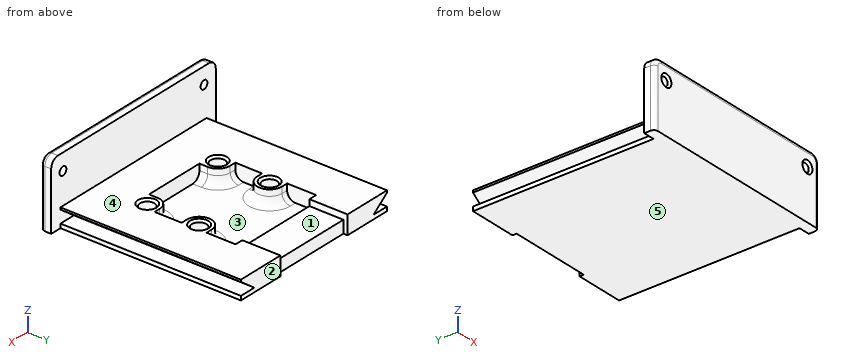
```python
from build123d import *

# Parameters (mm, degrees)
ESQUISSE1_W             = 43.5
ESQUISSE1_H             = 43.5
BOSS_EXTRU_1_DEPTH      = 3.5
ESQUISSE3_W             = 24
ESQUISSE3_H             = 24.5
ENL_V_MAT_EXTRU_1_DEPTH = 3.5
ENL_V_MAT_EXTRU_3_DEPTH = 43.5
ESQUISSE5_W             = 20
ESQUISSE5_H             = 9.18
ENL_V_MAT_EXTRU_4_DEPTH = 1.5
BOSS_EXTRU_2_DEPTH      = 3.5
ESQUISSE8_R             = 1.75
ENL_V_MAT_EXTRU_5_DEPTH = 3.5
ESQUISSE9_W             = 43.5
ESQUISSE9_H             = 43.5
BOSS_EXTRU_3_DEPTH      = 1
CONG_2_R                = 2
CHANFREIN1_SIZE         = 0.5
ESQUISSE10_W            = 20
ESQUISSE10_H            = 1
ENL_V_MAT_EXTRU_6_DEPTH = 3
ESQUISSE11_W            = 49
ESQUISSE11_H            = 16
BOSS_EXTRU_4_DEPTH      = 2.5
ESQUISSE12_R            = 1
ENL_V_MAT_EXTRU_7_DEPTH = 2.5
CONG_3_R                = 2
CONG_4_R                = 1
CHANFREIN2_SIZE         = 0.5


with BuildPart() as part:
    # Esquisse1 → Boss.-Extru.1 (new body)
    with BuildSketch(Plane.XY):
        with Locations((21.75, 21.75)):
            Rectangle(ESQUISSE1_W, ESQUISSE1_H)
    extrude(amount=BOSS_EXTRU_1_DEPTH)

    # Esquisse3 → Enlèv. mat.-Extru.1 (cut)
    with BuildSketch(Plane.XY.offset(3.5)):
        with Locations((21.75, 22.07)):
            Rectangle(ESQUISSE3_W, ESQUISSE3_H)
    extrude(amount=-ENL_V_MAT_EXTRU_1_DEPTH, mode=Mode.SUBTRACT)

    # Esquisse4 → Enlèv. mat.-Extru.3 (cut)
    with BuildSketch(Plane.XZ):
        Polygon((0, 0), (0, 3), (4, 0), align=None)
        Polygon((43.5, 3), (39.5, 0), (43.5, 0), align=None)
    extrude(amount=-ENL_V_MAT_EXTRU_3_DEPTH, mode=Mode.SUBTRACT)

    # Esquisse5 → Enlèv. mat.-Extru.4 (cut)
    with BuildSketch(Plane.XY.offset(3.5)):
        with Locations((21.75, 38.91)):
            Rectangle(ESQUISSE5_W, ESQUISSE5_H)
    extrude(amount=-ENL_V_MAT_EXTRU_4_DEPTH, mode=Mode.SUBTRACT)

    # Esquisse6 → Boss.-Extru.2 (add)
    with BuildSketch(Plane.XY.offset(3.5)):
        with BuildLine():
            Line((11.25, 27.32), (9.75, 27.32))
            Line((9.75, 27.32), (9.75, 21.32))
            Line((9.75, 21.32), (11.25, 21.32))
            ThreePointArc((11.25, 21.32), (14.25, 24.32), (11.25, 27.32))
        make_face()
        with BuildLine():
            Line((11.25, 14.82), (9.75, 14.82))
            Line((9.75, 14.82), (9.75, 9.82))
            Line((9.75, 9.82), (14.25, 9.82))
            Line((14.25, 9.82), (14.25, 11.82))
            ThreePointArc((14.25, 11.82), (13.371320344, 13.941320344), (11.25, 14.82))
        make_face()
        with BuildLine():
            Line((29.25, 11.82), (29.25, 9.82))
            Line((29.25, 9.82), (33.75, 9.82))
            Line((33.75, 9.82), (33.75, 14.82))
            Line((33.75, 14.82), (32.25, 14.82))
            ThreePointArc((32.25, 14.82), (30.128679656, 13.941320344), (29.25, 11.82))
        make_face()
        with BuildLine():
            Line((32.25, 27.32), (33.75, 27.32))
            Line((33.75, 27.32), (33.75, 21.32))
            Line((33.75, 21.32), (32.25, 21.32))
            ThreePointArc((32.25, 21.32), (29.25, 24.32), (32.25, 27.32))
        make_face()
    extrude(amount=-BOSS_EXTRU_2_DEPTH)

    # Esquisse8 → Enlèv. mat.-Extru.5 (cut)
    with BuildSketch(Plane.XY.offset(3.5)):
        with Locations((11.25, 24.32)):
            Circle(ESQUISSE8_R)
        with Locations((32.25, 24.32)):
            Circle(ESQUISSE8_R)
        with Locations((32.25, 11.82)):
            Circle(ESQUISSE8_R)
        with Locations((11.25, 11.82)):
            Circle(ESQUISSE8_R)
    extrude(amount=-ENL_V_MAT_EXTRU_5_DEPTH, mode=Mode.SUBTRACT)

    # Esquisse9 → Boss.-Extru.3 (add)
    with BuildSketch(Plane(origin=(0, 0, 0), x_dir=(-1, 0, 0), z_dir=(0, 0, -1))):
        with Locations((-21.75, 21.75)):
            Rectangle(ESQUISSE9_W, ESQUISSE9_H)
    extrude(amount=BOSS_EXTRU_3_DEPTH)

    # Congé2
    cong_2_edges = [part.edges().sort_by_distance(p)[0] for p in [
        (29.25, 24.32, 0),
        (33, 27.32, 0),
        (33, 21.32, 0),
        (14.25, 24.32, 0),
        (10.5, 21.32, 0),
        (10.5, 27.32, 0),
        (13.371320344, 13.941320344, 0),
        (14.25, 10.82, 0),
        (10.5, 14.82, 0),
        (30.128679656, 13.941320344, 0),
        (33, 14.82, 0),
        (29.25, 10.82, 0),
    ]]
    fillet(cong_2_edges, radius=CONG_2_R)

    # Chanfrein1
    chanfrein1_edges = [part.edges().sort_by_distance(p)[0] for p in [
        (9.5, 11.82, 3.5),
        (30.5, 11.82, 3.5),
        (30.5, 24.32, 3.5),
        (9.5, 24.32, 3.5),
    ]]
    chamfer(chanfrein1_edges, length=CHANFREIN1_SIZE)

    # Esquisse10 → Enlèv. mat.-Extru.6 (cut)
    with BuildSketch(Plane.XY.offset(2)):
        with Locations((21.75, 43)):
            Rectangle(ESQUISSE10_W, ESQUISSE10_H)
    extrude(amount=-ENL_V_MAT_EXTRU_6_DEPTH, mode=Mode.SUBTRACT)

    # Esquisse11 → Boss.-Extru.4 (add)
    with BuildSketch(Plane.XZ):
        with Locations((21.75, 7)):
            Rectangle(ESQUISSE11_W, ESQUISSE11_H)
    extrude(amount=BOSS_EXTRU_4_DEPTH)

    # Esquisse12 → Enlèv. mat.-Extru.7 (cut)
    with BuildSketch(Plane.XZ.offset(2.5)):
        with Locations(Location((0.75, 11, 0), (0, 0, 270))):
            Circle(ESQUISSE12_R)
        with Locations(Location((42.75, 11, 0), (0, 0, 270))):
            Circle(ESQUISSE12_R)
    extrude(amount=-ENL_V_MAT_EXTRU_7_DEPTH, mode=Mode.SUBTRACT)

    # Congé3
    cong_3_edges = [part.edges().sort_by_distance(p)[0] for p in [
        (-2.75, -1.25, 15),
        (46.25, -1.25, 15),
    ]]
    fillet(cong_3_edges, radius=CONG_3_R)

    # Congé4
    cong_4_edges = [part.edges().sort_by_distance(p)[0] for p in [
        (46.25, -2.5, 6),
        (-2.75, -2.5, 6),
        (21.75, -2.5, 15),
        (45.664213562, -2.5, 14.414213562),
        (-2.164213562, -2.5, 14.414213562),
    ]]
    fillet(cong_4_edges, radius=CONG_4_R)

    # Chanfrein2
    chanfrein2_edges = [part.edges().sort_by_distance(p)[0] for p in [
        (0.75, -2.5, 12),
        (42.75, -2.5, 12),
    ]]
    chamfer(chanfrein2_edges, length=CHANFREIN2_SIZE)


solid = part.part
```
Build history of the part. All positions in model axes, mm. Face numbers are marked on the shaded views. A direction names the side the tool comes from. Coordinates: 2 decimals unless noted, no trailing zeros. Write each loop counter-clockwise with the first axis right and the second up, starting at its lowest first coordinate (ties: lowest second). Pieces come first, ordered by that corner, then holes.
1. Band-saw the part on D-D, the plane y = 5. Give the cut face in (x, z).
Answer block:
outline: (0, -1) - (43.5, -1) - (43.5, 0) - (39.5, 0) - (43.5, 3) - (43.5, 3.5) - (0, 3.5) - (0, 3) - (4, 0) - (0, 0) - close
2. Pull direction Y, two halves, no side cores. Call the marked faces 1, 2 and 3: released by +Y, released by -Y, zero draft, split by the parting line, or undercut.
Answer block:
face 1: zero draft
face 2: released by +Y
face 3: undercut
3. 3-axis set-ups, long thin cutter, end or side, ignore diameter. For the marked faces 4 and 5: which of +Z, -Z, +X, -X, +Y, -Y reach the whole face in a straight line?
Answer block:
face 4: +Z, +X, -X, +Y
face 5: -Z, +X, -X, +Y, -Y
4. Band-saw the part on B-B, the plane x = 42.75. Give the cut face in (y, z).
Answer block:
outline: (-2.5, -1) - (43.5, -1) - (43.5, 0) - (0, 0) - (0, 2.44) - (43.5, 2.44) - (43.5, 3.5) - (0, 3.5) - (0, 10) - (-2, 10) - (-2.5, 9.5) - close; (-2.5, 12.5) - (-2, 12) - (0, 12) - (0, 15) - (-1.5, 15) arc R1 ccw to (-2.5, 14) - close
5. Drill centre lines: probe 1 along X at (y, z) = (-0.7, 11); probe 2 along Y at (x, z) = (32.25, 1.15); probe 3 along Y at (x, z) = (33, 1.25). Where is each one in solid material? Low to high.
Answer block:
probe 1: x = -2.75 to -0.25, 1.75 to 41.75, 43.75 to 46.25
probe 2: y = -2.5 to 10.07, 13.57 to 15.01, 21.13 to 22.57, 26.07 to 27.51, 34.32 to 43.5
probe 3: y = -2.5 to 10.24, 13.4 to 14.97, 21.17 to 22.74, 25.9 to 27.47, 34.32 to 43.5
6. Band-saw the part on A-A, the plane y = 24.32. Give the cut face in (x, z).
Answer block:
outline: (0, -1) - (43.5, -1) - (43.5, 0) - (39.5, 0) - (43.5, 3) - (43.5, 3.5) - (34.5, 3.5) - (34, 3) - (34, 0) - (30.5, 0) - (30.5, 3) - (30, 3.5) - (29.25, 3.5) - (29.25, 2) arc R2 cw to (27.25, 0) - (16.25, 0) arc R2 cw to (14.25, 2) - (14.25, 3.5) - (13.5, 3.5) - (13, 3) - (13, 0) - (9.5, 0) - (9.5, 3) - (9, 3.5) - (0, 3.5) - (0, 3) - (4, 0) - (0, 0) - close
7. Band-saw the part on C-C, the plane z = 8. Give the cut face in (x, y).
Answer block:
outline: (-2.75, -1.5) arc R1 ccw to (-1.75, -2.5) - (45.25, -2.5) arc R1 ccw to (46.25, -1.5) - (46.25, 0) - (-2.75, 0) - close
8. Drop flat-ended pins along their axis: pin 1 (2 mm diameter, centred on y = 31.5, z = 4, fed in from -X); pin 2 (1 mm diameter, centred on x = 32.5, y = 24.5, fed in from +Z); pin 3 (3 mm diameter, centred on x = 1.5, y = 20.5, fed in from +Z). Give the stop position or say it passes through.
Answer block:
pin 1: stops at x = 0
pin 2: stops at z = 0
pin 3: stops at z = 3.5
